```python
from build123d import *

# Parameters (mm, degrees)
F0_R     = 15.875
F1_DEPTH = 9.525
F2_R     = 8


with BuildPart() as f1:
    # F0 (on Top) → F1 (new body)
    with BuildSketch(Plane.XY):
        with BuildLine():
            ThreePointArc((-15.991178, -13.418191), (-20.875, 0), (-15.991178, 13.418191))
            Line((-15.991178, 13.418191), (-20.6832, 17.355265))
            ThreePointArc((-20.6832, 17.355265), (-32.626759, 12.588513), (-30, 0))
            ThreePointArc((-30, 0), (-32.626759, -12.588513), (-20.6832, -17.355265))
            Line((-20.6832, -17.355265), (-15.991178, -13.418191))
        make_face()
        with BuildLine():
            Line((-17.355265, 20.6832), (-13.418191, 15.991178))
            ThreePointArc((-13.418191, 15.991178), (-14.760854, 14.760854), (-15.991178, 13.418191))
            ThreePointArc((-15.991178, 13.418191), (-20.875, 0), (-15.991178, -13.418191))
            ThreePointArc((-15.991178, -13.418191), (-14.760854, -14.760854), (-13.418191, -15.991178))
            Line((-13.418191, -15.991178), (-17.355265, -20.6832))
            ThreePointArc((-17.355265, -20.6832), (-12.588513, -32.626759), (0, -30))
            ThreePointArc((0, -30), (12.588513, -32.626759), (17.355265, -20.6832))
            Line((17.355265, -20.6832), (13.418191, -15.991178))
            ThreePointArc((13.418191, -15.991178), (14.760854, -14.760854), (15.991178, -13.418191))
            Line((15.991178, -13.418191), (20.6832, -17.355265))
            ThreePointArc((20.6832, -17.355265), (32.626759, -12.588513), (30, 0))
            ThreePointArc((30, 0), (32.626759, 12.588513), (20.6832, 17.355265))
            Line((20.6832, 17.355265), (15.991178, 13.418191))
            ThreePointArc((15.991178, 13.418191), (14.760854, 14.760854), (13.418191, 15.991178))
            Line((13.418191, 15.991178), (17.355265, 20.6832))
            ThreePointArc((17.355265, 20.6832), (12.588513, 32.626759), (0, 30))
            ThreePointArc((0, 30), (-12.588513, 32.626759), (-17.355265, 20.6832))
        make_face()
        Circle(F0_R, mode=Mode.SUBTRACT)
    extrude(amount=F1_DEPTH)

    # F2
    f2_edges = [f1.edges().sort_by_distance(p)[0] for p in [
        (-20.6832, -17.355265, 4.7625),
        (20.6832, -17.355265, 4.7625),
        (17.355265, 20.6832, 4.7625),
        (20.6832, 17.355265, 4.7625),
        (-17.355265, -20.6832, 4.7625),
        (-20.6832, 17.355265, 4.7625),
        (-17.355265, 20.6832, 4.7625),
        (17.355265, -20.6832, 4.7625),
    ]]
    fillet(f2_edges, radius=F2_R)


solid = f1.part
```
Source: CAD feature listing. Evaluate the final solid. Frame: model axes, mm. A direction names the side the tool comes from. Round coordinates to 2 decimals unless told otherwise and drop trailing zeros. Write each loop counter-clockwise with the first axis right and the second up, starting at its lowest first coordinate (ties: lowest second). Pieces come first, ordered by that corner, then holes. Notation, with made-up numbers: M 87,54.25 L 145,54.25 A15 cw 145,80.25 Z; hole C 50.5,26 d6. An arc over 180 degrees is marked long. Use CSV: the item, a comma, the result in double quotes. Start each with the question number.
Q1. Cut plane D-D on x = -20. Output: boundary loops of the cut face in (y, z) (3 decimals), plus the area to 3 significant figures.
Q2. Cut plane B-B on y = 10. Output: boundary loops of the cut face in (x, z) (3 decimals).
Q3. Cut plane A-A on x = -3.5. Output: boundary loops of the cut face in (y, z) (3 decimals), plus the area to 3 significant figures.
Q4. First-contact query: P1, Ø4, axis at x = 9, z = 4, coming from the +Y side; P2, Ø1.5, axis at x = -14.5, z = 5, coming from the -Y side; P3, Ø2, axis at y = 3, z = 3, coming from the -X side; P4, Ø1, axis at y = 21, z = 8.5, coming from the -X side. Flat tips, straight axial feed; report the tip coordinate or a pass-through.
Q5. Access query for faces 4 (the face through (-17.53, -14.71, 4.7)), 5 (the face through (-17.54, 22.03, 4.83)). Directions: +Z, -Z, +X, -X, +Y, -Y. A direction counts if a zero-diameter tool reaches every point of the face in a straight line with its end or side. Return the directions, or none.
Q6. Pull-direction query (X, two-part tool) for faces 1 (the face through (-3.441, -15.497, 4.696)), 2 (the face through (15, -7, 9.525)), 3 (the face through (17.567, -22.129, 4.829)); classes: +X half, -X half, draft (parallel to the pull), parting line (faces both ways), or undercut.
Q7. Line query: line 1 (X direction, y = 16, z = 3.25); line 2 (Y direction, x = 17, z = 5.25); line 3 (X direction, y = -11.5, z = 1). Output: solid intervals per line, ascending. Write a range as from..to.
Results found:
1,outline,"M -16.663,0 L 16.663,0 L 16.663,9.525 L -16.663,9.525 Z"
1,area,"317 mm^2"
2,outline,"M -33.584,0 L -12.329,0 L -12.329,9.525 L -33.584,9.525 Z; M 12.329,0 L 33.584,0 L 33.584,9.525 L 12.329,9.525 Z"
3,outline,"M -32.816,0 L -15.484,0 L -15.484,9.525 L -32.816,9.525 Z; M 15.484,0 L 32.816,0 L 32.816,9.525 L 15.484,9.525 Z"
3,area,"330 mm^2"
4,P1,"y = 33.82"
4,P2,"y = -31.9"
4,P3,"x = -33.04"
4,P4,"x = -17.37"
5,face 4,"+Z, -Z"
5,face 5,"+Z, -Z, -X"
6,face 1,"undercut"
6,face 2,"draft"
6,face 3,"+X half"
7,line 1,"-29.62..-19.07, -13.43..13.43, 19.07..29.62"
7,line 2,"-27.87..-20.61, -14.26..14.26, 20.61..27.87"
7,line 3,"-33.13..-10.94, 10.94..33.13"
